Autodesk Inventor part; units mm, degrees
ref_plane "YZ Plane" through (0, 0, 0) normal (1, 0, 0) x (0, 1, 0)
ref_plane "XZ Plane" through (0, 0, 0) normal (0, 1, 0) x (-1, 0, 0)
ref_plane "XY Plane" through (0, 0, 0) normal (0, 0, 1) x (1, 0, 0)
sketch "Sketch1" plane through (0, 0, 0) normal (0, 0, 1) x (1, 0, 0)
  circle A0 centre (-3.0223, 127.0774) radius 1.5
  circle A1 centre (-3.0236, 60.0769) radius 1.5
  circle A2 centre (-3.0223, 127.0774) radius 1.5
  circle A3 centre (-3.0236, 60.0769) radius 1.5
  line L0 (3.5721, 158.6605) -> (3.572, -21.7605)
  line L1 (0.5721, 162.401) -> (0.572, -18.02)
  line L2 (0.572, 142.0774) -> (-14.428, 142.0774)
  line L3 (-29.428, 127.0774) -> (-29.428, 62.0774)
  line L4 (-14.428, 47.0774) -> (0.572, 47.0774)
  line L5 (0.572, 47.0774) -> (0.572, 142.0774)
  arc A4 (-14.428, 142.0774) -> (-29.428, 127.0774) centre (-14.428, 127.0774) ccw
  arc A5 (-29.428, 62.0774) -> (-14.428, 47.0774) centre (-14.428, 62.0774) ccw
  line L6 (-18.428, 119.5774) -> (-10.4279, 119.5774)
  line L7 (-4.428, 113.5774) -> (-4.428, 75.5774)
  line L8 (-10.428, 69.5774) -> (-18.428, 69.5774)
  line L9 (-24.428, 75.5774) -> (-24.428, 113.5774)
  arc A6 (-18.428, 119.5774) -> (-24.428, 113.5774) centre (-18.428, 113.5774) ccw
  arc A7 (-4.428, 113.5774) -> (-10.4279, 119.5774) centre (-10.4279, 113.5774) ccw
  arc A8 (-24.428, 75.5774) -> (-18.428, 69.5774) centre (-18.428, 75.5774) ccw
  arc A9 (-10.428, 69.5774) -> (-4.428, 75.5774) centre (-10.428, 75.5774) ccw
  line L10 (0.572, 142.0774) -> (3.572, 142.0774)
  line L11 (3.572, 142.0774) -> (3.572, 47.0774)
  line L12 (3.572, 47.0774) -> (0.572, 47.0774)
  line L13 (0.572, 47.0774) -> (0.572, 142.0774)
  point P0 (0, 0)
  point P1 (-29.428, 47.0774)
  point P2 (-29.428, 142.0774)
  point P3 (-24.428, 119.5774)
  point P4 (-4.428, 119.5774)
  point P5 (-24.428, 69.5774)
  point P6 (-24.428, 94.5774)
  point P7 (-29.428, 94.5774)
  point P8 (-14.428, 119.5774)
  point P9 (0.572, 47.0774)
  dimension "d0" = 3
  dimension "d1" = 30
  dimension "d2" = 95
  dimension "d3" = 15
  dimension "d4" = 15
  dimension "d7" = 50
  dimension "d8" = 20
  dimension "d9" = 6
  dimension "d10" = 95
extrude "Extrusion1" add sketch "Sketch1" along normal blind 2.5 contours L1 L4 A5 L3 A4 L2
sketch "Sketch2" plane through (0, 0, 2.5) normal (0, 0, 1) x (1, 0, 0)
  line L0 (0.572, 47.0774) -> (0.572, 142.0774)
  line L1 (0.572, 142.0774) -> (3.572, 142.0774)
  line L2 (3.572, 142.0774) -> (3.572, 47.0774)
  line L3 (3.572, 47.0774) -> (0.572, 47.0774)
  line L4 (0.572, 47.0774) -> (0.572, 142.0774)
  point P0 (0, 0)
  dimension "d13" = 3
extrude "Extrusion2" add sketch "Sketch2" along normal blind 15
fillet "Fillet1" radius 10 2 edges at (2.072, 47.0774, 17.5) (2.072, 142.0774, 17.5)
extrude "Extrusion3" add sketch "Sketch2" against normal blind 2.5
properties part number "screen_back_support_right"
Geometry: final body of the model. Coordinates: model frame, mm. A direction names the side the tool comes from. Coordinates: 2 decimals unless noted, no trailing zeros. Order: outer loops, then holes, each group sorted by start corner. A loop starts at its lowest first (then second) coordinate and runs counter-clockwise, first axis right, second up. Notation, with made-up numbers: M 2,35 L 23,35 A15 ccw 23,51 Z; hole C 45,-8 d6. An arc over 180 degrees is marked long. Answer in a Markdown table with one row per item. Add a question column.
Q1. Contact query for flat-ended pins moving along their axis: P1, Ø1.5, axis at y = 61, z = 7, coming from the -X side; P2, Ø15, axis at x = -16, y = 110.5, coming from the +Z side; P3, Ø0.8, axis at x = -15.5, z = 1, coming from the -Y side; P4, Ø3.5, axis at x = -3.02, y = 60.08, coming from the +Z side. Output: stop coordinate, or through.
Q2. Section query A-A on y = 74.5. Return the cut outline in (x, z).
Q3. Section query B-B on x = -2.5. Return the cut outline in (y, z).
Q4. Mould query, pull axis Y, two halves, no side actions, for faces 4 (the flat face through (-3, 47.077, 2)), 5 (the flat face through (0.572, 94, 10)), 6 (the cylindrical face through (-3.22, 58.59, 1.23)). Classes: released by +Y, released by -Y, zero draft, split by the parting line, or undercut.
Q5. Line query: L1, parallel to X at y = 104, z = 2.25; L2, parallel to Z at x = -4, y = 90; L3, parallel to X at y = 130, z = 10.25. Output: solid intervals per line, ascending.
Q6. Reachability of faces 1 (the cylindrical face through (-22.72, 117.77, 1.23)), 2 (the flat face through (-25, 95, 2.5)), 3 (the flat face through (2, 95, 17.5)) from +Z, -Z, +X, -X, +Y, -Y: full face, straight path, thin tool, end or side. Return the list, or none.
Q7. Section query C-C on x = -6.5. Return the cut outline in (y, z).
Q8. Section query D-D on y = 89. Return the cut outline in (x, z).
Completed:
| question | item | result |
|---|---|---|
| 1 | P1 | stops at x = 0.57 |
| 1 | P2 | passes through |
| 1 | P3 | stops at y = 47.09 |
| 1 | P4 | stops at z = 2.5 |
| 2 | outline | M -29.43,0 L -24.33,0 L -24.33,2.5 L -29.43,2.5 Z; M -4.53,0 L 3.57,0 L 3.57,17.5 L 0.57,17.5 L 0.57,2.5 L -4.53,2.5 Z |
| 3 | outline | M 47.08,0 L 58.67,0 L 58.67,2.5 L 47.08,2.5 Z; M 61.48,0 L 125.67,0 L 125.67,2.5 L 61.48,2.5 Z; M 128.48,0 L 142.08,0 L 142.08,2.5 L 128.48,2.5 Z |
| 4 | face 4 | released by -Y |
| 4 | face 5 | zero draft |
| 4 | face 6 | undercut |
| 5 | L1 | x = -29.43 to -24.43, -4.43 to 3.57 |
| 5 | L2 | z = 0 to 2.5 |
| 5 | L3 | x = 0.57 to 3.57 |
| 6 | face 1 | +Z, -Z |
| 6 | face 2 | +Z, -X, +Y, -Y |
| 6 | face 3 | +Z, +X, -X, +Y, -Y |
| 7 | outline | M 47.08,0 L 71.04,0 L 71.04,2.5 L 47.08,2.5 Z; M 118.11,0 L 142.08,0 L 142.08,2.5 L 118.11,2.5 Z |
| 8 | outline | M -29.43,0 L -24.43,0 L -24.43,2.5 L -29.43,2.5 Z; M -4.43,0 L 3.57,0 L 3.57,17.5 L 0.57,17.5 L 0.57,2.5 L -4.43,2.5 Z |
